Autodesk Inventor part; units mm, degrees
ref_plane "YZ Plane" through (0, 0, 0) normal (1, 0, 0) x (0, 1, 0)
ref_plane "XZ Plane" through (0, 0, 0) normal (0, 1, 0) x (-1, 0, 0)
ref_plane "XY Plane" through (0, 0, 0) normal (0, 0, 1) x (1, 0, 0)
sketch "Sketch1" plane through (0, 0, 0) normal (0, 0, 1) x (1, 0, 0)
  circle A0 centre (0, 0) radius 14.925 construction
  circle A1 centre (12.4625, 21.5857) radius 4
  circle A2 centre (-24.925, 0) radius 4
  circle A3 centre (12.4625, -21.5857) radius 4
  line L0 (12.4625, -21.5857) -> (12.4625, 21.5857) construction
  line L1 (12.4625, 21.5857) -> (-24.925, 0) construction
  line L2 (-24.925, 0) -> (12.4625, -21.5857) construction
  line L3 (12.4625, 21.5857) -> (7.4625, 12.9254) construction
  line L4 (-14.925, 0) -> (-24.925, 0) construction
  line L5 (12.4625, -21.5857) -> (7.4625, -12.9254) construction
  line L6 (80, 100) -> (-80, 100)
  line L7 (-100, 80) -> (-100, -80)
  line L8 (-80, -100) -> (80, -100)
  line L9 (100, -80) -> (100, 80)
  arc A4 (100, 80) -> (80, 100) centre (80, 80) ccw
  arc A5 (-80, 100) -> (-100, 80) centre (-80, 80) ccw
  arc A6 (-100, -80) -> (-80, -100) centre (-80, -80) ccw
  arc A7 (80, -100) -> (100, -80) centre (80, -80) ccw
  circle A8 centre (0, 0) radius 5
  point P0 (100, 100)
  point P1 (-100, -100)
  point P2 (-100, 100)
  dimension "d0" = 29.85
  dimension "d1" = 8
  dimension "d2" = 10
  dimension "d3" = 200
  dimension "d4" = 200
  dimension "d5" = 100
  dimension "d6" = 100
  dimension "d7" = 20
  dimension "d10" = 10
extrude "Extrusion1" add sketch "Sketch1" along normal blind 10
properties part number "Tractor_Static_4"
For this review, take the finished solid that the model builds, in its own axes (mm). Round coordinates to 2 decimals unless told otherwise and drop trailing zeros. Write each loop counter-clockwise with the first axis right and the second up, starting at its lowest first coordinate (ties: lowest second). Pieces come first, ordered by that corner, then holes. Notation, with made-up numbers: M 55.5,22 L 61.5,22 A16 cw 61.5,52 Z; hole C 26.25,-16 d7. An arc over 180 degrees is marked long. Write item = value, one per line. Start each with the question number.
(1) We need section B-B (x = 0). Give the boundary of the cut face in (y, z).
(2) The part is to be moulded in two halves that separate along Y. For faces 1 (the face through (100, -1, 5)), 2 (the face through (-94.297, 93.986, 4.93)), 3 (the face through (-1.08, 4.88, 4.93)), 4 (the face through (-28.92, -0.18, 4.93)), say which applies: +Y half, -Y half, draft (parallel to the pull), parting line (faces both ways), or undercut.
(3) We need section A-A (y = 0). Give the boundary of the cut face in (x, z) (3 decimals), then the cut area to 3 significant figures.
(4) Clearance check with a flat-ended pin moving along its axis: pin 1 Ø10.5 at (x, y) = (12.46, 21.59) entering from +Z. State where the tip first meets the part, or that it passes through.
(5) For line 1 along Y through (x, z) = (-25.5, 6.5); line 2 along X through (y, z) = (-0.5, 5); line 3 along Y through (x, z) = (14, 6), list the stretches that pass through material, from the lowest coordinate up.
Results found:
q1.outline = M -100,0 L -5,0 L -5,10 L -100,10 Z; M 5,0 L 100,0 L 100,10 L 5,10 Z
q2.face_1 = draft
q2.face_2 = +Y half
q2.face_3 = undercut
q2.face_4 = undercut
q3.outline = M -100,0 L -28.925,0 L -28.925,10 L -100,10 Z; M -20.925,0 L -5,0 L -5,10 L -20.925,10 Z; M 5,0 L 100,0 L 100,10 L 5,10 Z
q3.area = 1,820 mm²
q4.pin_1 = 10
q5.line_1 = -100 to -3.96, 3.96 to 100
q5.line_2 = -100 to -28.89, -20.96 to -4.97, 4.97 to 100
q5.line_3 = -100 to -25.28, -17.89 to 17.89, 25.28 to 100
